Autodesk Inventor part; units mm, degrees
ref_plane "YZ Plane" through (0, 0, 0) normal (1, 0, 0) x (0, 1, 0)
ref_plane "XZ Plane" through (0, 0, 0) normal (0, 1, 0) x (-1, 0, 0)
ref_plane "XY Plane" through (0, 0, 0) normal (0, 0, 1) x (1, 0, 0)
sketch "Sketch1" plane through (0, 0, 0) normal (0, 0, 1) x (1, 0, 0)
  line L0 (-17.8842, 30.4949) -> (102.1158, 30.4949)
  line L1 (102.1158, 30.4949) -> (102.1158, -89.5051)
  line L2 (102.1158, -89.5051) -> (-17.8842, -89.5051)
  line L3 (-17.8842, -89.5051) -> (-17.8842, 30.4949)
  line L4 (-17.8842, 30.4949) -> (87.1158, 30.4949)
  line L5 (87.1158, 30.4949) -> (87.1158, -74.5051)
  line L6 (87.1158, -74.5051) -> (-17.8842, -74.5051)
  line L7 (-17.8842, -74.5051) -> (-17.8842, 30.4949)
  point P0 (0, 0)
  point P1 (87.1158, 30.4949)
  point P2 (-17.8842, -74.5051)
  dimension "d0" = 120
  dimension "d1" = 120
  dimension "d2" = 105
  dimension "d3" = 105
extrude "Extrusion1" add sketch "Sketch1" along normal blind 1 contours L0 L1 L2 L3 L6 L5
properties part number "8006_Cu_groundplane_Tx_Filter_Stage2_MPSv2_v1" material "Copper"
Model file for the job. Use its own axes, mm. Round coordinates to 2 decimals unless told otherwise and drop trailing zeros. Loops run counter-clockwise (first coordinate to the right, second up) from the corner with the lowest first, then second, coordinate; pieces in that order, holes last.
1. Wall check: probe 1 along X at (y, z) = (-8.5, 0.9); probe 2 along Y at (x, z) = (0, 0.6). Give the ranges that are in metal, low to high.
Check values:
probe 1: x = 87.12 to 102.12
probe 2: y = -89.51 to -74.51
2. Band-saw the part on A-A, the plane z = 0.7. List the corners of the cut face in (x, y), and give its area (4 significant figures).
Check values:
outline: (-17.88, -89.51) - (102.12, -89.51) - (102.12, 30.49) - (87.12, 30.49) - (87.12, -74.51) - (-17.88, -74.51) - close
area: 3,375 mm2
3. Band-saw the part on B-B, the plane x = 84.5. List the corners of the cut face in (y, z).
Check values:
outline: (-89.51, 0) - (-74.51, 0) - (-74.51, 1) - (-89.51, 1) - close
4. Drop a flat-ended pin along its axis: P1, Ø0.5, axis at y = -34.5, z = 0.5, coming from the -X side. Give the stop position or say it passes through.
Check values:
P1: stops at x = 87.12
5. Band-saw the part on C-C, the plane y = -11. List the corners of the cut face in (x, z).
Check values:
outline: (87.12, 0) - (102.12, 0) - (102.12, 1) - (87.12, 1) - close
